Could you check a few things on this model? Use its own coordinates, in mm. Face numbers are marked on the shaded views. A direction names the side the tool comes from. Round coordinates to 2 decimals unless told otherwise and drop trailing zeros. Loops run counter-clockwise (first coordinate to the right, second up) from the corner with the lowest first, then second, coordinate; pieces in that order, holes last. Notation, with made-up numbers: M -26.5,89 L 4.5,89 A19 ccw 4.5,120 Z; hole C -32,-39 d3. An arc over 180 degrees is marked long. Answer in a Markdown table with one row per item.
Autodesk Fusion 360 part; units mm, degrees
sketch "Sketch1" plane through (0, 0, 0) normal (0, 0, 1) x (1, 0, 0)
  line L0 (0, 0) -> (8.5, 0)
  line L1 (8.5, 0) -> (8.5, 8.5)
  line L2 (8.5, 8.5) -> (0, 8.5)
  line L3 (0, 8.5) -> (0, 0)
  dimension "d1" = 8.5
extrude "Extrude1" add sketch "Sketch1" along normal blind 3
sketch "Sketch2" plane through (0, 0, 0) normal (0, 0, -1) x (1, 0, 0)
  line L0 (0, 0) -> (0, -8.5)
  line L1 (0, -8.5) -> (8.5, -8.5)
  line L2 (8.5, -8.5) -> (8.5, 0)
  line L3 (8.5, 0) -> (0, 0)
  line L4 (0.5, -0.5) -> (8, -0.5)
  line L5 (8, -0.5) -> (8, -8)
  line L6 (8, -8) -> (0.5, -8)
  line L7 (0.5, -8) -> (0.5, -0.5)
  line L8 (0.5, -0.5) -> (8, -8) construction
  line L9 (8.5, 0) -> (0, -8.5) construction
  dimension "d4" = 7.5
extrude "Extrude2" add sketch "Sketch2" along normal blind 29 contours L4 L5 L6 L7
sketch "Sketch3" plane through (8, 0, 0) normal (1, 0, 0) x (0, 1, 0)
  line L0 (8, 0) -> (0.5, 0)
  line L1 (0.5, 0) -> (0.5, -29)
  line L2 (0.5, -29) -> (8, -29)
  line L3 (8, -29) -> (8, 0)
  line L4 (0.5, -29) -> (4.25, -26.8349)
  line L5 (4.25, -26.8349) -> (8, -29)
  line L6 (8, -29) -> (0.5, -29)
  dimension "d7" = 120
extrude "Extrude3" cut sketch "Sketch3" against normal through all contours L2 L4 L5 L6
fillet "Fillet1" radius 1 2 edges at (4.25, 0.5, -29) (4.25, 8, -29)
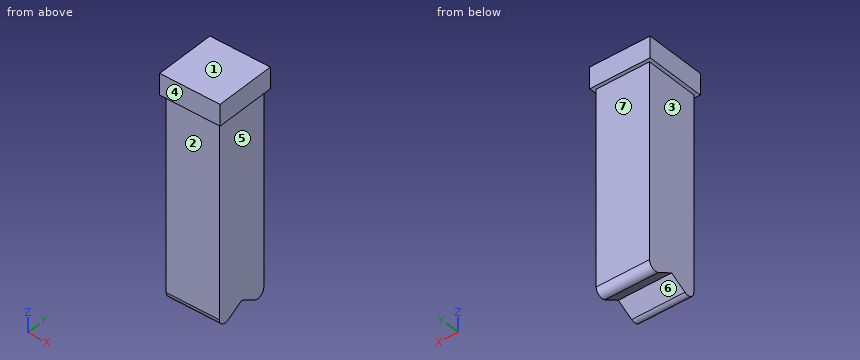
1) Will these pins go through, and if not, where does the flat tip stop? P1, Ø2, axis at x = 4, z = -15.5, coming from the -Y side; P2, Ø4, axis at x = 6, y = 2.5, coming from the -Z side; P3, Ø4, axis at y = 7.5, z = -22, coming from the -X side; P4, Ø5, axis at y = 7.5, z = -15.5, coming from the +X side.
Computed:
| item | result |
|---|---|
| P1 | stops at y = 0.5 |
| P2 | stops at z = -28.27 |
| P3 | stops at x = 0.5 |
| P4 | stops at x = 8 |
2) I want a section at C-C, the plane z = -3. Please give me the cut outline in (x, y), plus the area to 4 significant figures.
Computed:
| item | result |
|---|---|
| outline | M 0.5,0.5 L 8,0.5 L 8,8 L 0.5,8 Z |
| area | 56.25 mm² |
3) I want a section at A-A, the plane x = 3.25. Please give me the cut outline in (y, z), plus the area to 3 significant figures.
Computed:
| item | result |
|---|---|
| outline | M 0,0 L 0.5,0 L 0.5,-27.27 A1 ccw 2,-28.13 L 4.25,-26.83 L 6.5,-28.13 A1 ccw 8,-27.27 L 8,0 L 8.5,0 L 8.5,3 L 0,3 Z |
| area | 234 mm² |
4) If we mould it in two halves opening along Y, with no side actions, what happens to the marked faces 4, 5, 6 and 7? For each: released by +Y, released by -Y, zero draft, split by the parting line, or undercut.
Computed:
| item | result |
|---|---|
| face 4 | released by -Y |
| face 5 | zero draft |
| face 6 | undercut |
| face 7 | released by +Y |
5) I need wall thicknesses on line 1 (Y direction, x = 7, z = -6.5); line 2 (Z direction, x = 1.75, y = 5). Which ranges of each line are inside material? Lowest first, please.
Computed:
| item | result |
|---|---|
| line 1 | y = 0.5 to 8 |
| line 2 | z = -27.27 to 3 |
6) Which directions (+Z, -Z, +X, -X, +Y, -Y) give clear straight access to the entire face, cutting with the end or side of a thin tool? Please do the marked faces 1, 2 and 3.
Computed:
| item | result |
|---|---|
| face 1 | +Z, +X, -X, +Y, -Y |
| face 2 | -Z, +X, -X, -Y |
| face 3 | -Z, -X, +Y, -Y |
7) I want a section at B-B, the plane y = 1.5. Please give me the cut outline in (x, z).
Computed:
| item | result |
|---|---|
| outline | M 0,0 L 0.5,0 L 0.5,-28.27 L 8,-28.27 L 8,0 L 8.5,0 L 8.5,3 L 0,3 Z |
8) I want a section at D-D, the plane y = 5.25. Please give me the cut outline in (x, z).
Computed:
| item | result |
|---|---|
| outline | M 0,0 L 0.5,0 L 0.5,-27.41 L 8,-27.41 L 8,0 L 8.5,0 L 8.5,3 L 0,3 Z |
